Source: three-view drawing plus pictorial views. Frame: mm from the lowest corner of the part. A direction names the side the tool comes from. Give positions to 0.01 mm unless a question says otherwise; leave off trailing zeros. Order: outer loops, then holes, each group sorted by start corner. A loop starts at its lowest first (then second) coordinate and runs counter-clockwise, first axis right, second up.
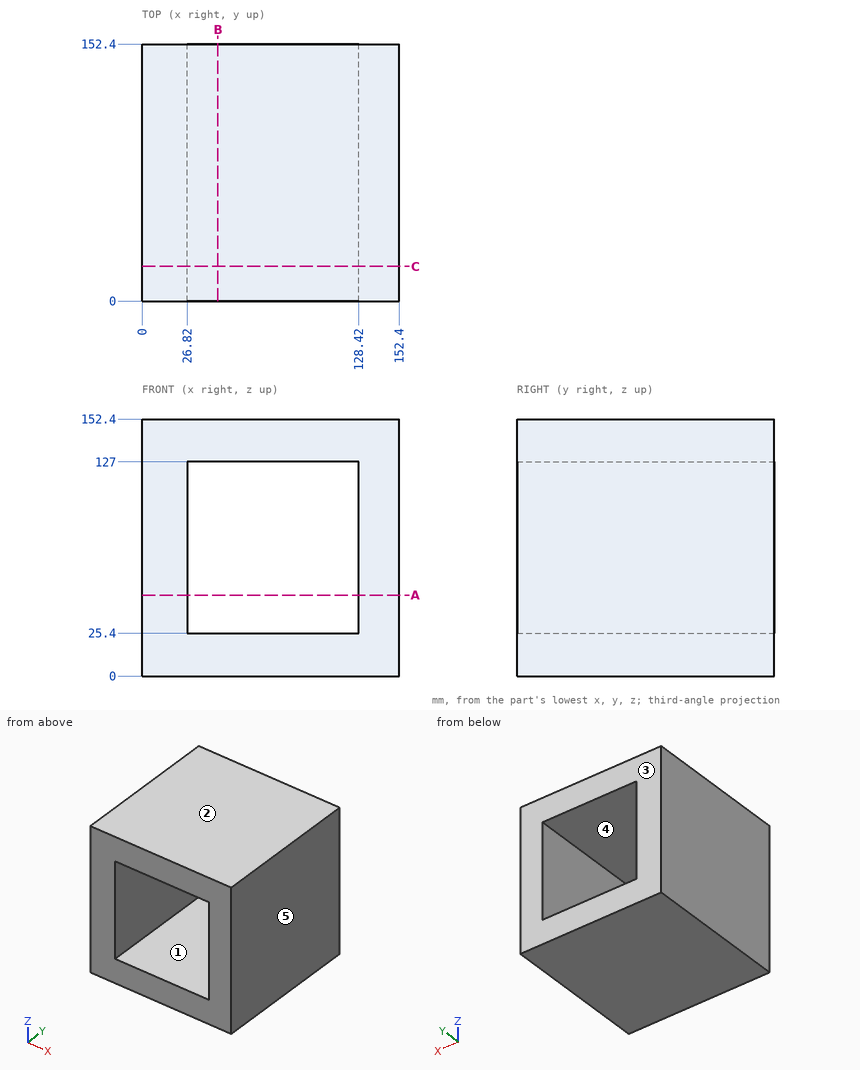
1) Section query A-A on z = 48. Output: boundary loops of the cut face in (x, y), and give its area (3 significant figures).
Checks:
outline: (0, 0) - (26.82, 0) - (26.82, 152.4) - (0, 152.4) - close; (128.42, 0) - (152.4, 0) - (152.4, 152.4) - (128.42, 152.4) - close
area: 7,740 mm2
2) Section query B-B on x = 45. Output: boundary loops of the cut face in (y, z), and give its area (3 significant figures).
Checks:
outline: (0, 0) - (152.4, 0) - (152.4, 25.4) - (0, 25.4) - close; (0, 127) - (152.4, 127) - (152.4, 152.4) - (0, 152.4) - close
area: 7,740 mm2
3) Pull-direction query (Z, two-part tool) for the marked faces 1, 2 and 3; classes: +Z half, -Z half, draft (parallel to the pull), parting line (faces both ways), or undercut.
Checks:
face 1: undercut
face 2: +Z half
face 3: draft
4) Ray query, L1, parallel to X at y = 94.5, z = 109.5; L2, parallel to Z at x = 46, y = 36.5. Return the intervals inside material, ascending.
Checks:
L1: x = 0 to 26.82, 128.42 to 152.4
L2: z = 0 to 25.4, 127 to 152.4
5) Section query C-C on y = 20.5. Output: boundary loops of the cut face in (x, z), and give its area (3 significant figures).
Checks:
outline: (0, 0) - (152.4, 0) - (152.4, 152.4) - (0, 152.4) - close; hole (26.82, 25.4) - (128.42, 25.4) - (128.42, 127) - (26.82, 127) - close
area: 12,900 mm2
6) Reachability of the marked faces 4 and 5 from +Z, -Z, +X, -X, +Y, -Y: full face, straight path, thin tool, end or side. Return the list, or none.
Checks:
face 4: +Y, -Y
face 5: +Z, -Z, +X, +Y, -Y
